```python
from build123d import *

# Parameters (mm, degrees)
DODANIE_WYCI_GNI_CIE1_DEPTH = 12.5
SKORUPA1_START              = 4
SKORUPA1_OUTLINE_W          = 27
SKORUPA1_OUTLINE_H          = 17
SKORUPA1_DEPTH              = 26
SZKIC2_R                    = 3
WYTNIJ_WYCI_GNI_CIE1_DEPTH  = 50
SZKIC3_R                    = 3
SZKIC3_R_2                  = 4
WYTNIJ_WYCI_GNI_CIE2_DEPTH  = 50
ZAOKR_GLENIE1_R             = 0.5


# Read off the part's stored shape, not the designer's step: Skorupa1
with BuildPart() as part:
    # Szkic1 → Dodanie-wyciągnięcie1 (new, symmetric)
    with BuildSketch(Plane(origin=(0, 0, 0), x_dir=(1, 0, 0), z_dir=(0, 1, 0))):
        Polygon((0, 0), (0, -30), (4, -30), (30, -4), (30, 0), align=None)
    extrude(amount=DODANIE_WYCI_GNI_CIE1_DEPTH, both=True)

    # Skorupa1 outline → Skorupa1 (cut)
    with BuildSketch(Plane.XY.offset(SKORUPA1_START)):
        with Locations((17.5, 0)):
            Rectangle(SKORUPA1_OUTLINE_W, SKORUPA1_OUTLINE_H)
    extrude(amount=SKORUPA1_DEPTH, mode=Mode.SUBTRACT)

    # Szkic2 → Wytnij-wyciągnięcie1 (cut)
    with BuildSketch(Plane(origin=(4, 0, 0), x_dir=(0, 0, -1), z_dir=(1, 0, 0))):
        with Locations((-20, 0)):
            Circle(SZKIC2_R)
    extrude(amount=-WYTNIJ_WYCI_GNI_CIE1_DEPTH, mode=Mode.SUBTRACT)

    # Szkic3 → Wytnij-wyciągnięcie2 (cut)
    with BuildSketch(Plane.XY.offset(4)):
        with Locations((20, 0)):
            Circle(SZKIC3_R)
        with Locations((18, 24.919871589)):
            Circle(SZKIC3_R_2)
    extrude(amount=-WYTNIJ_WYCI_GNI_CIE2_DEPTH, mode=Mode.SUBTRACT)

    # Zaokrąglenie1
    zaokr_glenie1_edges = [part.edges().sort_by_distance(p)[0] for p in [
        (17, -8.5, 4),
        (4, -8.5, 17),
        (4, 0, 4),
        (17, 8.5, 4),
        (4, 8.5, 17),
    ]]
    fillet(zaokr_glenie1_edges, radius=ZAOKR_GLENIE1_R)


solid = part.part
```
Geometry check sheet. Reference: the model listing, model coordinates, mm. A direction names the side the tool comes from. Coordinates: 2 decimals unless noted, no trailing zeros. Order: outer loops, then holes, each group sorted by start corner. A loop starts at its lowest first (then second) coordinate and runs counter-clockwise, first axis right, second up.
Q1. Sectioned sample at A-A on z = 20. Record the cut outline in (x, y), and give its area (3 significant figures).
Reply:
outline: (0, -12.5) - (14, -12.5) - (14, -8.5) - (4.5, -8.5) arc R0.5 cw to (4, -8) - (4, -3) - (0, -3) - close; (0, 3) - (4, 3) - (4, 8) arc R0.5 cw to (4.5, 8.5) - (14, 8.5) - (14, 12.5) - (0, 12.5) - close
area: 156 mm2
Q2. Sectioned sample at C-C on x = 20. Record the cut outline in (y, z), and give its area (3 significant figures).
Reply:
outline: (-12.5, 0) - (-3, 0) - (-3, 4) - (-8, 4) arc R0.5 cw to (-8.5, 4.5) - (-8.5, 14) - (-12.5, 14) - close; (3, 0) - (12.5, 0) - (12.5, 14) - (8.5, 14) - (8.5, 4.5) arc R0.5 cw to (8, 4) - (3, 4) - close
area: 156 mm2
Q3. Depth check by flat-ended pin: pin 1 Ø3 at (x, y) = (13, -4) entering from +Z; pin 2 Ø5 at (y, z) = (-1.5, 23.5) entering from +X; pin 3 Ø8 at (x, y) = (18, 5) entering from +Z. Enter the tip coordinate at first touch or a pass-through.
Reply:
pin 1: stops at z = 4
pin 2: stops at x = 4
pin 3: stops at z = 17.94
Q4. Draft check along Z on faces 1 (the face through (0, 0, 15)), 2 (the face through (2, 0, 23)), 3 (the face through (17, 11, 17)). Enter one of: released by +Z, released by -Z, zero draft, split by the parting line, or undercut.
Reply:
face 1: zero draft
face 2: undercut
face 3: released by +Z
Q5. Thickness scan on probe 1 along Y at (x, z) = (9, 23.5); probe 2 along Y at (x, z) = (20, 0.95); probe 3 along X at (y, z) = (3.25, 7). Record the ranges inside material, lowest first.
Reply:
probe 1: y = -12.5 to -8.5, 8.5 to 12.5
probe 2: y = -12.5 to -3, 3 to 12.5
probe 3: x = 0 to 4
Q6. Tool access check on faces 4 (the face through (2, 0, 30)), 5 (the face through (17, 2, 4)). Record the directions out of +Z, -Z, +X, -X, +Y, -Y that give a thin tool (end or side, any length) a straight path to the whole face; none if there is none.
Reply:
face 4: +Z, +X, -X, +Y, -Y
face 5: +Z, +X
Q7. Sectioned sample at B-B on y = 0. Record the cut outline in (x, z).
Reply:
outline: (0, 0) - (17, 0) - (17, 4) - (4.5, 4) arc R0.5 cw to (4, 4.5) - (4, 17) - (0, 17) - close; (0, 23) - (4, 23) - (4, 30) - (0, 30) - close; (23, 0) - (30, 0) - (30, 4) - (23, 4) - close
Q8. Sectioned sample at D-D on z = 7. Record the cut outline in (x, y), and give its area (3 significant figures).
Reply:
outline: (0, -12.5) - (27, -12.5) - (27, -8.5) - (4.5, -8.5) arc R0.5 cw to (4, -8) - (4, 8) arc R0.5 cw to (4.5, 8.5) - (27, 8.5) - (27, 12.5) - (0, 12.5) - close
area: 284 mm2
